Drawing for the job (mm, zero at the part's lowest x, y, z). A direction names the side the tool comes from. Coordinates: 2 decimals unless noted, no trailing zeros. Write each loop counter-clockwise with the first axis right and the second up, starting at its lowest first coordinate (ties: lowest second). Pieces come first, ordered by that corner, then holes. Notation, with made-up numbers: M -34.75,-22.5 L 8.25,-22.5 A32 cw 8.25,15.5 Z; hole C 52,73.5 d4. An arc over 180 degrees is marked long. Put each result on its own line as item: value. Start each with the question number.
Q1. Which spindle directions (+Z, -Z, +X, -X, +Y, -Y) get a long thin tool onto all of the face, cutting with end or side? Do the marked faces 1, 2 and 3. Say none if no direction does.
Q2. Cut at A-A (z = 20.5). Write the cut outline in (x, y), then the cut area to 3 significant figures.
Q3. Cut at B-B (x = 85). Write the cut outline in (y, z), then the cut area to 4 significant figures.
Q4. Drill centre lines: line 1 along Y through (x, z) = (206, 1.7); line 2 along X through (y, z) = (91, 1.15); line 3 along Y through (x, z) = (155, 17.5). Where is each one in solid material? Low to high.
Q5. Pull direction Y, two halves, no side cores. Call the marked faces 4, 5 and 6: pulls with the +Y half, pulls with the -Y half, needs draft (parallel to the pull), parting line crosses it, or undercut.
Q6. Drop flat-ended pins along their axis: pin 1 (10 mm diameter, centred on y = 52.5, z = 11.5, fed in from +X); pin 2 (1.5 mm diameter, centred on x = 157, z = 15, fed in from +Y); pin 3 (1.2 mm diameter, centred on y = 86, z = 16, fed in from -X). Give the stop position or say it passes through.
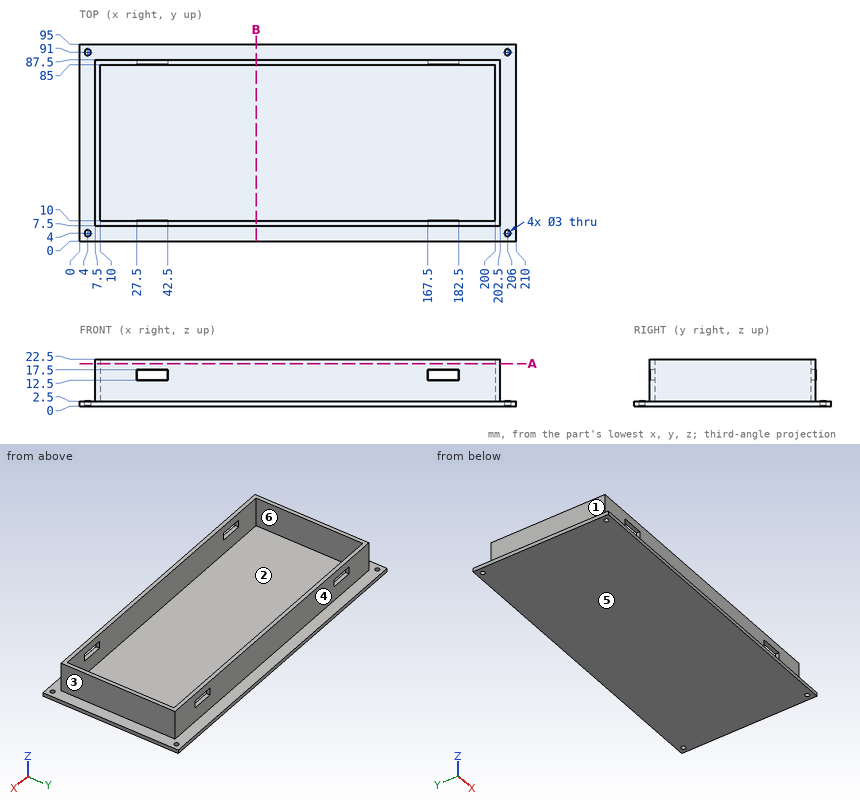
Computed values:
1. face 1: +Z, -X, +Y, -Y
1. face 2: +Z
1. face 3: +Z, +X, +Y, -Y
2. outline: M 7.5,7.5 L 202.5,7.5 L 202.5,87.5 L 7.5,87.5 Z; hole M 10,10 L 200,10 L 200,85 L 10,85 Z
2. area: 1,350 mm2
3. outline: M 0,0 L 95,0 L 95,2.5 L 87.5,2.5 L 87.5,22.5 L 85,22.5 L 85,2.5 L 10,2.5 L 10,22.5 L 7.5,22.5 L 7.5,2.5 L 0,2.5 Z
3. area: 337.5 mm2
4. line 1: 0 to 2.5, 5.5 to 89.5, 92.5 to 95
4. line 2: 0 to 2.5, 5.5 to 204.5, 207.5 to 210
4. line 3: 7.5 to 10, 85 to 87.5
5. face 4: pulls with the +Y half
5. face 5: needs draft
5. face 6: undercut
6. pin 1: x = 202.5
6. pin 2: y = 87.5
6. pin 3: x = 7.5
